The listing builds one solid part. Answer for the finished solid, in the listing's coordinates (mm). Give positions to 0.01 mm unless a question says otherwise; leave off trailing zeros. Order: outer loops, then holes, each group sorted by start corner. A loop starts at its lowest first (then second) coordinate and runs counter-clockwise, first axis right, second up.
Autodesk Inventor part; units mm, degrees
ref_plane "YZ Plane" through (0, 0, 0) normal (1, 0, 0) x (0, 1, 0)
ref_plane "XZ Plane" through (0, 0, 0) normal (0, 1, 0) x (-1, 0, 0)
ref_plane "XY Plane" through (0, 0, 0) normal (0, 0, 1) x (1, 0, 0)
sketch "Sketch1" plane through (0, 0, 0) normal (0, 0, 1) x (1, 0, 0)
  line L0 (4.5, -29.1615) -> (4.5, -46.55)
  line L1 (4.5, -46.55) -> (13, -46.55)
  arc A0 (13, -46.55) -> (15, -44.55) centre (13, -44.55) ccw
  line L2 (15, -44.55) -> (15, -15.75)
  line L3 (15, -15.75) -> (45, -15.75)
  line L4 (45, 39.4571) -> (45, -15.75)
  line L5 (-45, -15.75) -> (-45, 39.4571)
  line L6 (-45, -15.75) -> (-15, -15.75)
  line L7 (-15, -15.75) -> (-15, -44.55)
  arc A1 (-15, -44.55) -> (-13, -46.55) centre (-13, -44.55) ccw
  line L8 (-13, -46.55) -> (-4.5, -46.55)
  line L9 (-4.5, -46.55) -> (-4.5, -29.1615)
  line L10 (-4.5, -29.1615) -> (4.5, -29.1615)
  circle A2 centre (7.5, -43.35) radius 1.75
  circle A3 centre (7.5, -25.35) radius 1.75
  circle A4 centre (-7.5, -25.35) radius 1.75
  circle A5 centre (-7.5, -43.35) radius 1.75
  line L11 (45, 39.4571) -> (-45, 39.4571)
  line L12 (-23.9404, 34.5074) -> (-20.8237, 34.5074)
  ellipse E0 centre (-19.8512, 32.8923) end of major axis (-19.8512, 35.0136) minor radius 1.5 (-18.8787, 34.5074) -> (-20.8237, 34.5074) ccw
  line L13 (-18.8787, 34.5074) -> (-15.7619, 34.5074)
  line L14 (-15.7619, 34.5074) -> (-15.7619, 27.8723)
  line L15 (-15.7619, 27.8723) -> (-23.9404, 27.8723)
  line L16 (-23.9404, 27.8723) -> (-23.9404, 34.5074)
  line L17 (15.7619, 34.5074) -> (18.8787, 34.5074)
  ellipse E1 centre (19.8512, 32.8923) end of major axis (19.8512, 35.0136) minor radius 1.5 (20.8237, 34.5074) -> (18.8787, 34.5074) ccw
  line L18 (20.8237, 34.5074) -> (23.9404, 34.5074)
  line L19 (23.9404, 34.5074) -> (23.9404, 27.8723)
  line L20 (23.9404, 27.8723) -> (15.7619, 27.8723)
  line L21 (15.7619, 27.8723) -> (15.7619, 34.5074)
  point P0 (0, 0)
extrude "Extrusion1" add sketch "Sketch1" along normal blind 2 contours L10 L9 L8 A1 L7 L6 L5 L11 L4 L3 L2 A0 L1 L0 | L12 E0 L13 L14 L15 L16 | L17 E1 L18 L19 L20 L21
properties part number "lead" material "Lead"
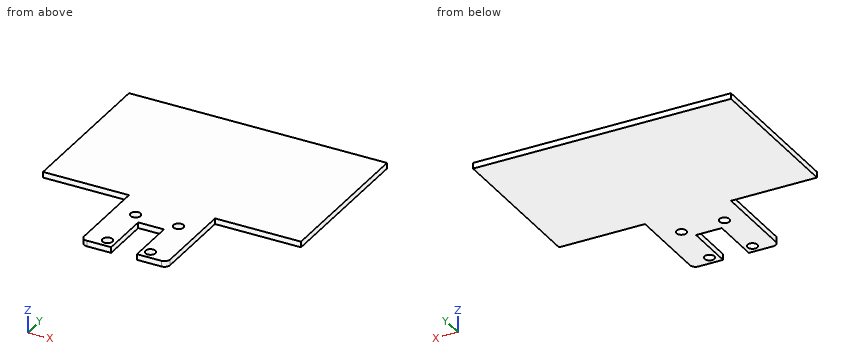
1) Given P1, Ø1, axis at x = -29, z = 0.5, coming from the -Y side; P2, Ø1, axis at y = -41.5, z = 1, coming from the +X side, each flat-ended and moving along its own axis, determine where each tip first touches the part or whether it passes through.
Geometry says:
P1: stops at y = -15.75
P2: stops at x = 15
2) Find section B-B (y = -43.35). Write down the section's boundary in (x, z).
Geometry says:
outline: (-15, 0) - (-9.25, 0) - (-9.25, 2) - (-15, 2) - close; (-5.75, 0) - (-4.5, 0) - (-4.5, 2) - (-5.75, 2) - close; (4.5, 0) - (5.75, 0) - (5.75, 2) - (4.5, 2) - close; (9.25, 0) - (15, 0) - (15, 2) - (9.25, 2) - close
3) Find section D-D (z = 0.9). Write down the section's boundary in (x, y), then the cut area to 3 significant figures.
Geometry says:
outline: (-45, -15.75) - (-15, -15.75) - (-15, -44.55) arc R2 ccw to (-13, -46.55) - (-4.5, -46.55) - (-4.5, -29.16) - (4.5, -29.16) - (4.5, -46.55) - (13, -46.55) arc R2 ccw to (15, -44.55) - (15, -15.75) - (45, -15.75) - (45, 39.46) - (-45, 39.46) - close; hole circle Ø3.5 at (-7.5, -43.35); hole circle Ø3.5 at (-7.5, -25.35); hole circle Ø3.5 at (7.5, -43.35); hole circle Ø3.5 at (7.5, -25.35)
area: 5,700 mm2
4) Find section A-A (x = -7.5). Write down the section's boundary in (y, z).
Geometry says:
outline: (-46.55, 0) - (-45.1, 0) - (-45.1, 2) - (-46.55, 2) - close; (-41.6, 0) - (-27.1, 0) - (-27.1, 2) - (-41.6, 2) - close; (-23.6, 0) - (39.46, 0) - (39.46, 2) - (-23.6, 2) - close
5) Find section C-C (y = -25.35). Write down the section's boundary in (x, z).
Geometry says:
outline: (-15, 0) - (-9.25, 0) - (-9.25, 2) - (-15, 2) - close; (-5.75, 0) - (5.75, 0) - (5.75, 2) - (-5.75, 2) - close; (9.25, 0) - (15, 0) - (15, 2) - (9.25, 2) - close
6) Straight lines are drawn through the part: probe 1 along Y at (x, z) = (7.5, 0.7); probe 2 along X at (y, z) = (-22.5, 1.75); probe 3 along Y at (x, z) = (-20, 1.35). For each, find the intervals that lie inside material, in ascending order.
Geometry says:
probe 1: y = -46.55 to -45.1, -41.6 to -27.1, -23.6 to 39.46
probe 2: x = -15 to 15
probe 3: y = -15.75 to 39.46
